Geometry: see drawing. Coordinates: mm, zero at the bounding-box minimum. A direction names the side the tool comes from. Give positions to 0.01 mm unless a question says otherwise; leave off trailing zeros. Loops run counter-clockwise (first coordinate to the right, second up) from the corner with the lowest first, then second, coordinate; pieces in that order, holes last. Notation, with made-up numbers: M -2.5,50.5 L 23.5,50.5 A22 ccw 23.5,88.5 Z; hole C 19.5,-23.5 d9. An arc over 180 degrees is marked long. Put each result on its own line as item: value.
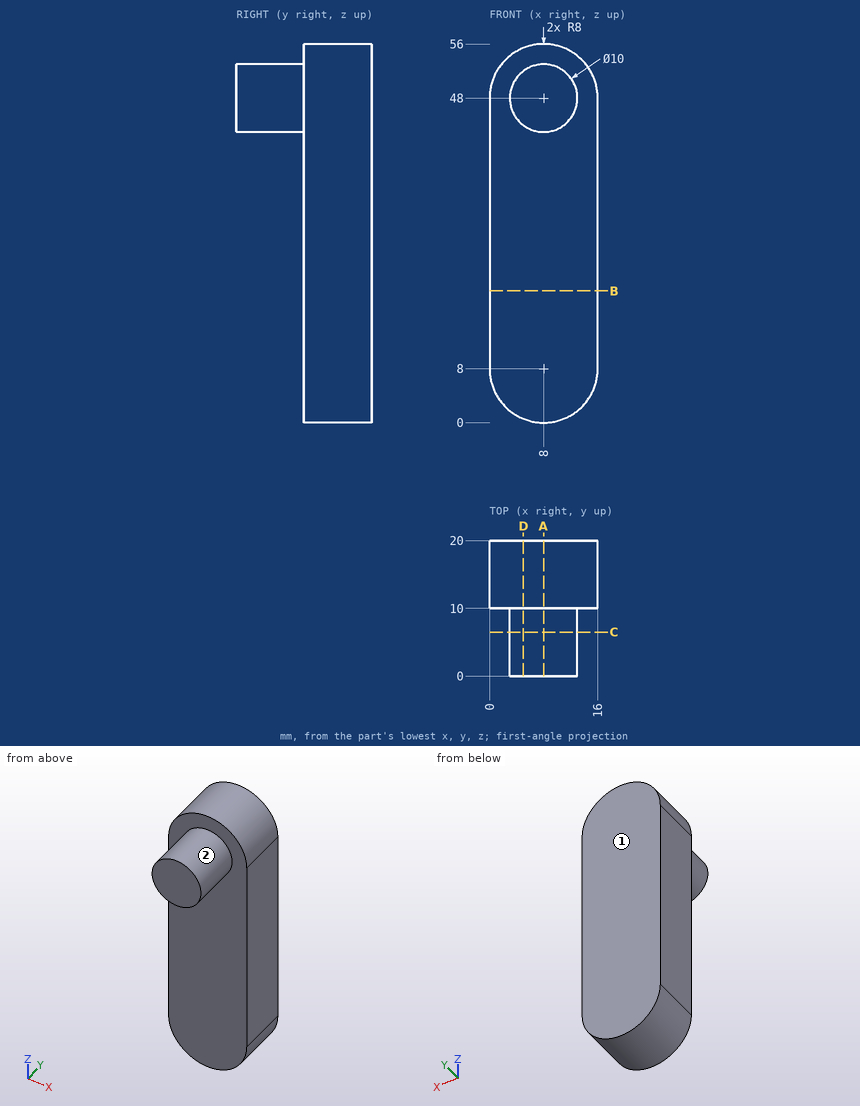
1. Section query C-C (y = 6.5). Output: boundary loops of the cut face in (x, z).
Found:
outline: C 8,48 d10
2. Section query D-D (x = 5). Output: boundary loops of the cut face in (y, z).
Found:
outline: M 0,44 L 10,44 L 10,0.58 L 20,0.58 L 20,55.42 L 10,55.42 L 10,52 L 0,52 Z
3. Material intervals for line 1 (Y direction, x = 1, z = 50.5); line 2 (Z direction, x = 7.75, y = 18.75); line 3 (Z direction, x = 14.25, y = 12.75), sorted ascending. Write a range as from..to.
Found:
line 1: 10..20
line 2: 0..56
line 3: 3.01..52.99
4. Section query A-A (x = 8). Output: boundary loops of the cut face in (y, z), plus the area to 3 significant figures.
Found:
outline: M 0,43 L 10,43 L 10,0 L 20,0 L 20,56 L 10,56 L 10,53 L 0,53 Z
area: 660 mm^2
5. Section query B-B (z = 19.5). Output: boundary loops of the cut face in (x, y), plus the area to 3 significant figures.
Found:
outline: M 0,10 L 16,10 L 16,20 L 0,20 Z
area: 160 mm^2
6. Access query for the marked faces 1 and 2. Directions: +Z, -Z, +X, -X, +Y, -Y. A direction counts if a zero-diameter tool reaches every point of the face in a straight line with its end or side. Return the directions, or none.
Found:
face 1: +Z, -Z, +X, -X, +Y
face 2: -Y
7. Contact query for flat-ended pins moving along their axis: P1, Ø1.5, axis at x = 4.5, y = 17.5, coming from the +Z side; P2, Ø2, axis at x = 14, y = 10.5, coming from the -Z side (3 decimals); P3, Ø1.5, axis at x = 9, z = 5.5, coming from the -Y side. Output: stop coordinate, or through.
Found:
P1: z = 55.51
P2: z = 1.755
P3: y = 10
